```python
from build123d import *

# Parameters (mm, degrees)
SKETCH1_R               = 4.25
SKETCH1_R_2             = 2.1
BOSS_EXTRUDE1_DEPTH     = 5
SKETCH2_W               = 23
SKETCH2_H               = 60
CUT_EXTRUDE1_DEPTH      = 10
FILLET1_R               = 5
FILLET2_R               = 5
ESQUISSE1_W             = 61.110635513
ESQUISSE1_H             = 10.431484261
ENL_V_MAT_EXTRU_1_DEPTH = 10
ESQUISSE5_W             = 55
ESQUISSE5_H             = 5
BOSS_EXTRU_3_DEPTH      = 20
BOSS_EXTRU_3_DEPTH_BACK = 9
ESQUISSE6_W             = 55
ESQUISSE6_H             = 28
BOSS_EXTRU_4_DEPTH      = 4
CONG_2_R                = 10
ESQUISSE11_R            = 2.5
ENL_V_MAT_EXTRU_2_DEPTH = 4


with BuildPart() as part:
    # Sketch1 → Boss-Extrude1 (new body)
    with BuildSketch(Plane.XY):
        with BuildLine():
            Line((-50.417601538, -29.831415105), (-27.417601538, -29.831415105))
            ThreePointArc((-27.417601538, -29.831415105), (0.082398462, -23.727510052), (27.582398462, -29.831415105))
            Line((27.582398462, -29.831415105), (50.582398462, -29.831415105))
            Line((50.582398462, -29.831415105), (50.582398462, 25.168584895))
            ThreePointArc((50.582398462, 25.168584895), (49.117932367, 28.704118801), (45.582398462, 30.168584895))
            Line((45.582398462, 30.168584895), (-45.417601538, 30.168584895))
            ThreePointArc((-45.417601538, 30.168584895), (-48.953135444, 28.704118801), (-50.417601538, 25.168584895))
            Line((-50.417601538, 25.168584895), (-50.417601538, -29.831415105))
        make_face()
        with Locations((12.582398462, -0.519851907)):
            Circle(SKETCH1_R, mode=Mode.SUBTRACT)
        with Locations((10.082398462, -13.519851907)):
            Circle(SKETCH1_R_2, mode=Mode.SUBTRACT)
        with Locations((-9.917601538, -13.519851907)):
            Circle(SKETCH1_R_2, mode=Mode.SUBTRACT)
        with Locations((-12.417601538, -0.519851907)):
            Circle(SKETCH1_R, mode=Mode.SUBTRACT)
        with Locations((-9.917601538, 12.480148093)):
            Circle(SKETCH1_R_2, mode=Mode.SUBTRACT)
        with Locations((10.082398462, 12.480148093)):
            Circle(SKETCH1_R_2, mode=Mode.SUBTRACT)
    extrude(amount=BOSS_EXTRUDE1_DEPTH)

    # Sketch2 → Cut-Extrude1 (cut)
    with BuildSketch(Plane.XY.offset(5)):
        with Locations((-38.917601538, 0.168584895)):
            Rectangle(SKETCH2_W, SKETCH2_H)
        with Locations((39.082398462, 0.168584895)):
            Rectangle(SKETCH2_W, SKETCH2_H)
    extrude(amount=-CUT_EXTRUDE1_DEPTH, mode=Mode.SUBTRACT)

    # Fillet1
    fillet1_edges = [part.edges().sort_by_distance(p)[0] for p in [
        (27.582398462, 30.168584895, 2.5),
    ]]
    fillet(fillet1_edges, radius=FILLET1_R)

    # Fillet2
    fillet2_edges = [part.edges().sort_by_distance(p)[0] for p in [
        (-27.417601538, 30.168584895, 2.5),
    ]]
    fillet(fillet2_edges, radius=FILLET2_R)

    # Esquisse1 → Enlèv. mat.-Extru.1 (cut)
    with BuildSketch(Plane.XY.offset(5)):
        with Locations((0.082398462, -28.943252183)):
            Rectangle(ESQUISSE1_W, ESQUISSE1_H)
    extrude(amount=-ENL_V_MAT_EXTRU_1_DEPTH, mode=Mode.SUBTRACT)

    # Esquisse5 → Boss.-Extru.3 (add, two sides)
    with BuildSketch(Plane(origin=(0, 30.168584895, 0), x_dir=(1, 0, 0), z_dir=(0, 1, 0))) as boss_extru_3_sk:
        with Locations((0.082398462, -2.5)):
            Rectangle(ESQUISSE5_W, ESQUISSE5_H)
    extrude(amount=BOSS_EXTRU_3_DEPTH)
    extrude(boss_extru_3_sk.sketch, amount=-BOSS_EXTRU_3_DEPTH_BACK)

    # Esquisse6 → Boss.-Extru.4 (add)
    with BuildSketch(Plane(origin=(0, 50.168584895, 0), x_dir=(1, 0, 0), z_dir=(0, 1, 0))):
        with Locations((0.082398462, -14)):
            Rectangle(ESQUISSE6_W, ESQUISSE6_H)
    extrude(amount=BOSS_EXTRU_4_DEPTH)

    # Congé2
    cong_2_edges = [part.edges().sort_by_distance(p)[0] for p in [
        (0.082398462, 50.168584895, 5),
        (0.082398462, 54.168584895, 0),
    ]]
    fillet(cong_2_edges, radius=CONG_2_R)

    # Esquisse11 → Enlèv. mat.-Extru.2 (cut)
    with BuildSketch(Plane(origin=(0, 54.168584895, 0), x_dir=(1, 0, 0), z_dir=(0, 1, 0))):
        with Locations((-24.5, -24.42)):
            Circle(ESQUISSE11_R)
        with Locations((24.5, -24.42)):
            Circle(ESQUISSE11_R)
        with BuildLine():
            Line((-19, -19.5), (19, -19.5))
            ThreePointArc((19, -19.5), (19.707106781, -19.792893219), (20, -20.5))
            Line((20, -20.5), (20, -40.5))
            Line((20, -40.5), (-20, -40.5))
            Line((-20, -40.5), (-20, -20.5))
            ThreePointArc((-20, -20.5), (-19.707106781, -19.792893219), (-19, -19.5))
        make_face()
    extrude(amount=-ENL_V_MAT_EXTRU_2_DEPTH, mode=Mode.SUBTRACT)


solid = part.part
```
Check sheet for the modelled part. Datum: model origin and axes. Units: mm. A direction names the side the tool comes from. Give positions to 0.01 mm unless a question says otherwise; leave off trailing zeros. Order: outer loops, then holes, each group sorted by start corner. A loop starts at its lowest first (then second) coordinate and runs counter-clockwise, first axis right, second up. Notation, with made-up numbers: (39.25, 17.25) -> (89.25, 17.25) arc R16 cw to (89.25, 48.25) -> close; hole circle Ø4 at (8.5, -30). An arc over 180 degrees is marked (long way). Return JSON: item names as keys, results as strings.
1. Go/stop test with flat-tipped pins: P1, Ø2, axis at x = 6.5, y = 52.5, coming from the +Z side; P2, Ø6, axis at x = -24.5, z = 24.42, coming from the -Y side; P3, Ø5.5, axis at x = -9.92, y = -13.52, coming from the +Z side. Record where each tip stops, or that it passes through.
From the geometry:
{"P1": "z = 19.5", "P2": "y = 50.17", "P3": "z = 5"}
2. Set-up check for faces 1 (the flat face through (27.582, 21, 4)), 2 (the flat face through (0, 50.169, 19)), 3 (the flat face through (-20, 52, 24)): record each of +Z, -Z, +X, -X, +Y, -Y from which the full face is reachable in a straight line by a thin tool's end or side.
From the geometry:
{"face 1": "+Z, -Z, +X, +Y, -Y", "face 2": "+Z, +X, -X, -Y", "face 3": "+Z, +Y, -Y"}
3. Material ranges on probe 1 along X at (y, z) = (53.35, 24.42); probe 2 along Y at (x, z) = (14, 15); probe 3 along Z at (x, y) = (-22, 32), recorded low to high. Write a range as [from, to].
From the geometry:
{"probe 1": "[-27.42, -27], [-22, -20], [20, 22], [27, 27.58]", "probe 2": "[50.17, 54.17]", "probe 3": "[0, 5]"}
4. Mould release check, pull along Y, two halves, no side actions. Record for faces 4 (the cylindrical face through (0.47, 51.16, 2.85)), 5 (the cylindrical face through (-8.364, 0.757, 2.465)), 6 (the flat face through (0, -23.728, 3)): +Y half, -Y half, draft (parallel to the pull), parting line (faces both ways), or undercut.
From the geometry:
{"face 4": "+Y half", "face 5": "undercut", "face 6": "-Y half"}
5. Cross-section at C-C, the plane z = 2.75. Record the cut outline in (x, y).
From the geometry:
{"outline": "(-27.42, -23.73) -> (27.58, -23.73) -> (27.58, 51.06) -> (-27.42, 51.06) -> close; hole circle Ø8.5 at (-12.42, -0.52); hole circle Ø4.2 at (-9.92, -13.52); hole circle Ø4.2 at (-9.92, 12.48); hole circle Ø4.2 at (10.08, -13.52); hole circle Ø4.2 at (10.08, 12.48); hole circle Ø8.5 at (12.58, -0.52)"}
6. Cross-section at A-A, the plane x = -23. Record the cut outline in (y, z).
From the geometry:
{"outline": "(-23.73, 0) -> (44.17, 0) arc R10 ccw to (54.17, 10) -> (54.17, 22.42) -> (50.17, 22.42) -> (50.17, 15) arc R10 cw to (40.17, 5) -> (-23.73, 5) -> close; (50.17, 26.42) -> (54.17, 26.42) -> (54.17, 28) -> (50.17, 28) -> close"}
7. Cross-section at D-D, the plane x = -1.5. Record the cut outline in (y, z).
From the geometry:
{"outline": "(-23.73, 0) -> (44.17, 0) arc R10 ccw to (54.17, 10) -> (54.17, 19.5) -> (50.17, 19.5) -> (50.17, 15) arc R10 cw to (40.17, 5) -> (-23.73, 5) -> close"}
8. Cross-section at B-B, the plane z = 24.42. Record the cut outline in (x, y), plus the area to 3 significant figures.
From the geometry:
{"outline": "(-27.42, 50.17) -> (-27, 50.17) -> (-27, 54.17) -> (-27.42, 54.17) -> close; (-22, 50.17) -> (-20, 50.17) -> (-20, 54.17) -> (-22, 54.17) -> close; (20, 50.17) -> (22, 50.17) -> (22, 54.17) -> (20, 54.17) -> close; (27, 50.17) -> (27.58, 50.17) -> (27.58, 54.17) -> (27, 54.17) -> close", "area": "20.0 mm^2"}
